Check sheet for the modelled part. Datum: model origin and axes. Units: mm. Round coordinates to 2 decimals unless told otherwise and drop trailing zeros. Order: outer loops, then holes, each group sorted by start corner. A loop starts at its lowest first (then second) coordinate and runs counter-clockwise, first axis right, second up. Notation, with made-up numbers: M 2,-9 L 32,-9 A17 ccw 32,21 Z; hole C -3.5,26 d1. An arc over 180 degrees is marked long. One line per item, written item: value. Start each with the question number.
(1) Cross-section at B-B, the plane z = 56.25. Enter the section's corners in (x, y), and give its area (3 significant figures).
(2) Depth check by flat-ended pin: pin 1 Ø4.5 at (x, z) = (8.75, -56.25) entering from +Y. Enter the tip coordinate at first touch or a pass-through.
(3) Thickness scan on L1, parallel to Z at x = -8.75, y = 1.5; L2, parallel to Z at x = 9.5, y = 1.4. Record the ranges inside material, lowest first.
(4) Cross-section at C-C, the plane y = 1.9. Enter the section's corners in (x, z), and give its area (3 significant figures).
(5) Cross-section at A-A, the plane x = 8.75. Enter the section's corners in (y, z).
(6) Release check for a two-part mould opening along Z. For faces 1 (the face through (9.29, 1.48, -53.81)), 2 (the face through (0, 1, 65)), 3 (the face through (0, 1, -65)), 4 (the face through (0, 0, 1)) record: released by +Z, released by -Z, zero draft, split by the parting line, or undercut.
Autodesk Inventor part; units mm, degrees
ref_plane "YZ Plane" through (0, 0, 0) normal (1, 0, 0) x (0, 1, 0)
ref_plane "XZ Plane" through (0, 0, 0) normal (0, 1, 0) x (-1, 0, 0)
ref_plane "XY Plane" through (0, 0, 0) normal (0, 0, 1) x (1, 0, 0)
sketch "Sketch1" plane through (0, 0, 0) normal (0, 1, 0) x (-1, 0, 0)
  line L0 (17.5, 65) -> (-17.5, 65)
  line L1 (-17.5, 65) -> (-17.5, -65)
  line L2 (-17.5, -65) -> (17.5, -65)
  line L3 (17.5, -65) -> (17.5, 65)
  line L4 (17.5, 65) -> (-17.5, -65) construction
  line L5 (-17.5, 65) -> (17.5, -65) construction
  line L6 (-17.5, 65) -> (0, 65)
  line L7 (0, 65) -> (0, 47.5)
  line L8 (0, 47.5) -> (-17.5, 47.5)
  line L9 (-17.5, 47.5) -> (-17.5, 65)
  line L10 (17.5, 65) -> (0, 65)
  line L11 (0, 65) -> (0, 47.5)
  line L12 (0, 47.5) -> (17.5, 47.5)
  line L13 (17.5, 47.5) -> (17.5, 65)
  line L14 (17.5, -65) -> (0, -65)
  line L15 (0, -65) -> (0, -47.5)
  line L16 (0, -47.5) -> (17.5, -47.5)
  line L17 (17.5, -47.5) -> (17.5, -65)
  line L18 (0, -47.5) -> (-17.5, -47.5)
  line L19 (-17.5, -47.5) -> (-17.5, -65)
  line L20 (-17.5, -65) -> (0, -65)
  line L21 (0, -65) -> (0, -47.5)
  circle A0 centre (8.75, 56.25) radius 2.5
  circle A1 centre (-8.75, 56.25) radius 2.5
  circle A2 centre (8.75, -56.25) radius 2.5
  circle A3 centre (-8.75, -56.25) radius 2.5
  point P0 (0, 0)
  dimension "d0" = 35
  dimension "d1" = 130
  dimension "d2" = 17.5
  dimension "d3" = 17.5
  dimension "d4" = 17.5
  dimension "d5" = 17.5
  dimension "d6" = 5
  dimension "d7" = 5
  dimension "d8" = 5
  dimension "d9" = 5
  dimension "d10" = 17.5
  dimension "d11" = 17.5
  dimension "d12" = 8.75
  dimension "d13" = 8.75
  dimension "d14" = 8.75
  dimension "d15" = 8.75
  dimension "d16" = 8.75
  dimension "d17" = 8.75
extrude "Extrusion1" add sketch "Sketch1" along normal blind 3
properties part number "cap"
Values found:
1. outline: M -17.5,0 L -11.25,0 L -11.25,3 L -17.5,3 Z; M -6.25,0 L 6.25,0 L 6.25,3 L -6.25,3 Z; M 11.25,0 L 17.5,0 L 17.5,3 L 11.25,3 Z
1. area: 75.0 mm^2
2. pin 1: through
3. L1: -65 to -58.75, -53.75 to 53.75, 58.75 to 65
3. L2: -65 to -58.63, -53.87 to 53.87, 58.63 to 65
4. outline: M -17.5,-65 L 17.5,-65 L 17.5,65 L -17.5,65 Z; hole C -8.75,-56.25 d5; hole C -8.75,56.25 d5; hole C 8.75,-56.25 d5; hole C 8.75,56.25 d5
4. area: 4,470 mm^2
5. outline: M 0,-65 L 3,-65 L 3,-58.75 L 0,-58.75 Z; M 0,-53.75 L 3,-53.75 L 3,53.75 L 0,53.75 Z; M 0,58.75 L 3,58.75 L 3,65 L 0,65 Z
6. face 1: undercut
6. face 2: released by +Z
6. face 3: released by -Z
6. face 4: zero draft
